Verification items for the finished model (mm, model axes). A direction names the side the tool comes from. Give positions to 0.01 mm unless a question says otherwise; leave off trailing zeros. Order: outer loops, then holes, each group sorted by start corner. A loop starts at its lowest first (then second) coordinate and runs counter-clockwise, first axis right, second up.
(1) Mould release check, pull along Y, two halves, no side actions. Record for faces 1 (the face through (123, 3, -37)), 2 (the face through (127.286, 1.282, -56.89)), 3 (the face through (113.918, -9.364, -36.814)): pulls with the +Y half, pulls with the -Y half, needs draft (parallel to the pull), parting line crosses it, or undercut.
(2) Gauge pin test, flat ends, axial feed: pin 1 (3 mm diameter, centred on y = -7.5, z = -38.5, fed in from -X); pin 2 (10 mm diameter, centred on y = 2, z = -68, fed in from +X); pin 3 (8 mm diameter, centred on x = 63.5, z = -55, fed in from -Y). Record the tip position at first contact, or that the pin passes through.
(3) Access from +Z, -Z, +X, -X, +Y, -Y to the whole of each face (thin tool, end or side, straight path). Record for faces 4 (the face through (122.51, 5.54, -41.26)), 5 (the face through (123, 2.6, -58)), 6 (the face through (123, -10, -52.411)), 7 (the face through (117, 4, -64.411)).
(4) Scan lines: L1, parallel to Y at x = 119, z = -27.5; L2, parallel to Y at x = 97.5, z = -57; L3, parallel to X at y = -16, z = -44. Record each from-to range of solid material in increasing order.
(5) Sectioned sample at D-D on x = 57. Record the cut outline in (y, z).
(6) Sectioned sample at A-A on y = -9.5. Record the cut outline in (x, z), plus the area to 3 significant figures.
(7) Sectioned sample at B-B on y = -3.5. Record the cut outline in (x, z), plus the area to 3 significant figures.
(8) Sectioned sample at C-C on z = -31.5. Record the cut outline in (x, y).
```python
from build123d import *

# Parameters (mm, degrees)
SKETCH2_R           = 1.5
BOSS_EXTRUDE1_DEPTH = 8
SKETCH11_W          = 24.345630124
SKETCH11_H          = 31
BOSS_EXTRUDE4_DEPTH = 30
SKETCH12_W          = 25
SKETCH12_H          = 25
CUT_EXTRUDE7_DEPTH  = 14.34563
CUT_EXTRUDE8_REACH  = 26.346
SKETCH13_R          = 3.1
SKETCH14_R          = 5
CUT_EXTRUDE9_DEPTH  = 5.5
SKETCH15_R          = 1.6
CUT_EXTRUDE10_DEPTH = 5.5
CUT_EXTRUDE11_REACH = 32
SKETCH16_R          = 1.6
CUT_EXTRUDE12_DEPTH = 2.6
FILLET2_R           = 3


with BuildPart() as part:
    # Sketch2 → Boss-Extrude1 (new body)
    with BuildSketch(Plane(origin=(0, 0, 0), x_dir=(1, 0, 0), z_dir=(0, 1, 0))):
        with BuildLine():
            Line((-38.837197709, 64.4109018), (-14.876439197, 64.4109018))
            Line((-14.876439197, 64.4109018), (-6.491567585, 70.282052109))
            Line((-6.491567585, 70.282052109), (-6.491567585, 77.282052109))
            Line((-6.491567585, 77.282052109), (13.508432415, 77.282052109))
            Line((13.508432415, 77.282052109), (13.508432415, 70.282052109))
            Line((13.508432415, 70.282052109), (21.893304027, 64.4109018))
            Line((21.893304027, 64.4109018), (45.85406254, 64.4109018))
            Line((45.85406254, 64.4109018), (45.85406254, 52.4109018))
            Line((45.85406254, 52.4109018), (17.508432415, 52.4109018))
            ThreePointArc((17.508432415, 52.4109018), (3.508432415, 58.207416665), (-10.491567585, 52.4109018))
            Line((-10.491567585, 52.4109018), (-38.837197709, 52.4109018))
            Line((-38.837197709, 52.4109018), (-38.837197709, 64.4109018))
        make_face()
        with Locations((-32.991567585, 58.4109018)):
            Circle(SKETCH2_R, mode=Mode.SUBTRACT)
        with Locations((40.008432415, 58.4109018)):
            Circle(SKETCH2_R, mode=Mode.SUBTRACT)
    extrude(amount=BOSS_EXTRUDE1_DEPTH)

    # Sketch11 → Boss-Extrude4 (add)
    with BuildSketch(Plane(origin=(0, 8, 0), x_dir=(-1, 0, 0), z_dir=(0, -1, 0))):
        with Locations((26.664382647, 39.9109018)):
            Rectangle(SKETCH11_W, SKETCH11_H)
    extrude(amount=BOSS_EXTRUDE4_DEPTH)

    # Sketch12 → Cut-Extrude7 (cut)
    with BuildSketch(Plane.ZY.offset(38.837197709)):
        with Locations((-39.9109018, -9.5)):
            Rectangle(SKETCH12_W, SKETCH12_H)
    extrude(amount=-CUT_EXTRUDE7_DEPTH, mode=Mode.SUBTRACT)

    # Sketch13 → Cut-Extrude8 (cut, up to next)
    with BuildSketch(Plane(origin=(-14.491567585, 0, 0), x_dir=(0, 0, -1), z_dir=(1, 0, 0)), mode=Mode.PRIVATE) as cut_extrude8_sk1:
        with Locations((39.9109018, -9.5)):
            Circle(SKETCH13_R)
    cut_extrude8_tool1 = extrude(cut_extrude8_sk1.sketch, amount=-CUT_EXTRUDE8_REACH, mode=Mode.PRIVATE) & part.part
    add(cut_extrude8_tool1.solids().sort_by_distance((-14.491568, -9.5, -39.910902))[0], mode=Mode.SUBTRACT)

    # Sketch14 → Cut-Extrude9 (cut)
    with BuildSketch(Plane(origin=(-14.491567585, 0, 0), x_dir=(0, 0, -1), z_dir=(1, 0, 0))):
        with Locations((39.9109018, -9.5)):
            Circle(SKETCH14_R)
    extrude(amount=-CUT_EXTRUDE9_DEPTH, mode=Mode.SUBTRACT)

    # Sketch15 → Cut-Extrude10 (cut)
    with BuildSketch(Plane.XY.offset(-24.4109018)):
        with Locations((-31.664382647, -9.5)):
            Circle(SKETCH15_R)
    extrude(amount=-CUT_EXTRUDE10_DEPTH, mode=Mode.SUBTRACT)

    # Sketch16 → Cut-Extrude11 (cut, up to next)
    with BuildSketch(Plane(origin=(0, 8, 0), x_dir=(1, 0, 0), z_dir=(0, 1, 0)), mode=Mode.PRIVATE) as cut_extrude11_sk1:
        with Locations((-31.664382647, 39.9109018)):
            Circle(SKETCH16_R)
    cut_extrude11_tool1 = extrude(cut_extrude11_sk1.sketch, amount=-CUT_EXTRUDE11_REACH, mode=Mode.PRIVATE) & part.part
    add(cut_extrude11_tool1.solids().sort_by_distance((-31.664383, 8, -39.910902))[0], mode=Mode.SUBTRACT)

    # Sketch17 → Cut-Extrude12 (cut)
    with BuildSketch(Plane.XZ):
        Polygon((-31.259516777, -61.4109018), (-29.52746597, -58.4109018), (-31.259516777, -55.4109018), (-34.723618392, -55.4109018), (-36.4556692, -58.4109018), (-34.723618392, -61.4109018), align=None)
        Polygon((38.276381608, -61.4109018), (41.740483223, -61.4109018), (43.47253403, -58.4109018), (41.740483223, -55.4109018), (38.276381608, -55.4109018), (36.5443308, -58.4109018), align=None)
    extrude(amount=-CUT_EXTRUDE12_DEPTH, mode=Mode.SUBTRACT)

    # Fillet2
    fillet2_edges = [part.edges().sort_by_distance(p)[0] for p in [
        (-38.837197709, 4, -64.4109018),
        (-6.491567585, 4, -77.282052109),
        (13.508432415, 4, -77.282052109),
        (45.85406254, 4, -64.4109018),
        (45.85406254, 4, -52.4109018),
        (-14.491567585, 4, -52.4109018),
        (-14.491567585, -7, -24.4109018),
    ]]
    fillet(fillet2_edges, radius=FILLET2_R)


with BuildPart() as body_2:
    # Mirror2: mirrored copy
    add(part.part.mirror(Plane(origin=(45.85406254, 8, -64.4109018), x_dir=(0, 0, 1), z_dir=(-1, 0, 0))))


solid = body_2.part
```
Ans:
1. face 1: pulls with the -Y half
1. face 2: needs draft
1. face 3: undercut
2. pin 1: stops at x = 111.7
2. pin 2: stops at x = 130.09
2. pin 3: stops at y = 0
3. face 4: +Y, -Y
3. face 5: -Y
3. face 6: +X, -Y
3. face 7: -Z, +X, +Y, -Y
4. L1: y = 3 to 8
4. L2: y = 0 to 8
4. L3: x = 106.2 to 116.2
5. outline: (0, -64.41) - (8, -64.41) - (8, -52.41) - (0, -52.41) - close
6. outline: (106.2, -55.41) - (130.55, -55.41) - (130.55, -52.41) - (116.2, -52.41) - (116.2, -43.01) - (111.7, -43.01) - (111.7, -44.91) - (106.2, -44.91) - close; (106.2, -34.91) - (111.7, -34.91) - (111.7, -36.81) - (116.2, -36.81) - (116.2, -27.41) - (121.77, -27.41) - (121.77, -24.41) - (109.2, -24.41) arc R3 ccw to (106.2, -27.41) - close; (124.97, -27.41) - (130.55, -27.41) - (130.55, -24.41) - (124.97, -24.41) - close
6. area: 302 mm2
7. outline: (106.2, -55.41) - (130.55, -55.41) - (130.55, -52.41) - (116.2, -52.41) - (116.2, -27.41) - (130.55, -27.41) - (130.55, -24.41) - (109.2, -24.41) arc R3 ccw to (106.2, -27.41) - close
7. area: 394 mm2
8. outline: (106.2, -22) - (116.2, -22) - (116.2, 3) - (130.55, 3) - (130.55, 8) - (106.2, 8) - close
